Could you check a few things on this model? Use its own coordinates, in mm. Round coordinates to 2 decimals unless told otherwise and drop trailing zeros. Order: outer loops, then holes, each group sorted by start corner. A loop starts at its lowest first (then second) coordinate and runs counter-clockwise, first axis right, second up. Notation, with made-up numbers: (-3, 0.5) - (39, 0.5) arc R33 ccw to (39, 28.5) - close; hole circle Ø1 at (79, 32). An arc over 180 degrees is marked (long way). Return JSON: item names as keys, results as strings. Group by question number.
from build123d import *

# Parameters (mm, degrees)
DELKA_DEPTH       = 250
D_RA1_D           = 3.5
D_RA1_CBORE_D     = 6
D_RA1_CBORE_DEPTH = 3.5
LINPOLE1_COUNT    = 12
LINPOLE1_PITCH    = 20


with BuildPart() as part:
    # Skica1 → Delka (new body)
    with BuildSketch(Plane(origin=(0, 0, 0), x_dir=(1, 0, 0), z_dir=(0, 1, 0))):
        with BuildLine():
            Line((-4.1, -6.500009514), (4.1, -6.500009514))
            Line((4.1, -6.500009514), (4.5, -6.100009514))
            Line((4.5, -6.100009514), (4.5, -5.453944278))
            ThreePointArc((4.5, -5.453944278), (4.150323615, -5.260214834), (3.904469431, -4.945))
            Line((3.904469431, -4.945), (3.3, -4.890009514))
            Line((3.3, -4.890009514), (3.3, -4.110009514))
            Line((3.3, -4.110009514), (3.909510964, -4.045014121))
            ThreePointArc((3.909510964, -4.045014121), (4.154592253, -3.736176828), (4.5, -3.546074751))
            Line((4.5, -3.546074751), (4.5, -0.4))
            Line((4.5, -0.4), (4.1, 0))
            Line((4.1, 0), (-1.4, 0))
            ThreePointArc((-1.4, 0), (-1.8, -0.2), (-2.2, 0))
            Line((-2.2, 0), (-4.1, 0))
            Line((-4.1, 0), (-4.5, -0.4))
            Line((-4.5, -0.4), (-4.5, -3.546074751))
            ThreePointArc((-4.5, -3.546074751), (-4.154592253, -3.736176828), (-3.909510964, -4.045014121))
            Line((-3.909510964, -4.045014121), (-3.3, -4.110009514))
            Line((-3.3, -4.110009514), (-3.3, -4.890009514))
            Line((-3.3, -4.890009514), (-3.904469431, -4.945))
            ThreePointArc((-3.904469431, -4.945), (-4.150323615, -5.260214834), (-4.5, -5.453944278))
            Line((-4.5, -5.453944278), (-4.5, -6.100009514))
            Line((-4.5, -6.100009514), (-4.1, -6.500009514))
        make_face()
    extrude(amount=DELKA_DEPTH)

    # Díra1 (through all)
    with Locations(Plane.XY.offset(6.500009514)):
        with Locations((0, 15)):
            d_ra1 = CounterBoreHole(D_RA1_D / 2, D_RA1_CBORE_D / 2, D_RA1_CBORE_DEPTH)

    # Zkosení1: read off the stored shape, not the designer's step
    # Zkosení1 outline → Zkosení1 (revolve, cut)
    with BuildSketch(Plane.XZ.offset(-15)):
        Polygon((2.050000176, -1.76e-07), (1.75, 0.3), (1.75, -1.76e-07), align=None)
        Polygon((3, 6.500009514), (3, 6.200009514), (3.3, 6.500009514), align=None)
    zkosen_1 = revolve(axis=Axis((0, 15, 0), (0, 0, 1)), mode=Mode.SUBTRACT)

    # LinPole1: Díra1, Zkosení1 ×12
    with Locations(*[(0, i * LINPOLE1_PITCH, 0) for i in range(1, LINPOLE1_COUNT)]):
        add(d_ra1, mode=Mode.SUBTRACT)
        add(zkosen_1, mode=Mode.SUBTRACT)


solid = part.part
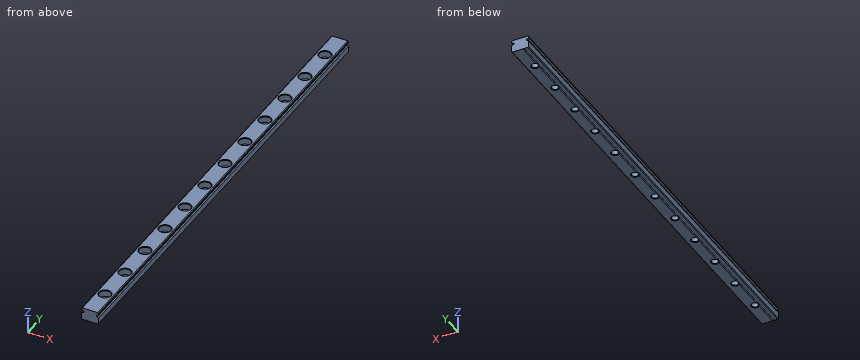
1) I want a section at B-B, the plane z = 2. Give the number of separate pieces and of enclosed holes in the cut face, plus the area to 3 significant figures.
2) Will this pin go through, and if not, where does the flat tip stop? pin 1 (1.8 mm diameter, centred on x = -1, y = 75.5, fed in from +Z).
3) If I drill on line 1 along Z through (x, y) = (-3.5, 16.5); line 2 along X through (y, z) = (235, 2.1); line 3 along X through (y, z) = (236, 1), over which ranges is the centre line in solid material (lowest first)? Write a range as from..to.
4) I want a section at A-A, the plane y = 83. List the corners of the cut face in (x, z) for me (3 decimals).
Outcome:
{
 "1": {"separate pieces": "1", "enclosed holes": "12", "area": "2,130 mm^2"},
 "2": {"pin 1": "z = 3"},
 "3": {"line 1": "0..4.09, 4.91..6.5", "line 2": "-4.5..-1.75, 1.75..4.5", "line 3": "-4.5..-1.44, 1.44..4.5"},
 "4": {"outline": "(-4.5, 0.4) - (-4.1, 0) - (-2.2, 0) arc R0.5 cw to (-1.4, 0) - (4.1, 0) - (4.5, 0.4) - (4.5, 3.546) arc R1 cw to (3.91, 4.045) - (3.3, 4.11) - (3.3, 4.89) - (3.904, 4.945) arc R1 cw to (4.5, 5.454) - (4.5, 6.1) - (4.1, 6.5) - (-4.1, 6.5) - (-4.5, 6.1) - (-4.5, 5.454) arc R1 cw to (-3.904, 4.945) - (-3.3, 4.89) - (-3.3, 4.11) - (-3.91, 4.045) arc R1 cw to (-4.5, 3.546) - close"}
}
